from build123d import *

# Parameters (mm, degrees)
F0_R     = 5.25
F1_DEPTH = 5.5
F3_DEPTH = 6
F5_DEPTH = 6
F7_DEPTH = 6
F8_R     = 5


with BuildPart() as f1:
    # F0 (on Right) → F1 (new body)
    with BuildSketch(Plane.YZ):
        Polygon((76, -45), (76, 45), (-66, 45), (-66, 40), (-76, 40), (-76, -45), align=None)
        with Locations((-30, -25)):
            Circle(F0_R, mode=Mode.SUBTRACT)
        with Locations((-30, 26)):
            Circle(F0_R, mode=Mode.SUBTRACT)
    extrude(amount=F1_DEPTH)

    # F2 (on face) → F3 (join)
    with BuildSketch(Plane(origin=(0, 76, 0), x_dir=(-1, 0, 0), z_dir=(0, 1, 0))):
        with BuildLine():
            Line((110.5, 45), (0, 45))
            Line((0, 45), (0, -45))
            Line((0, -45), (81.5, -45))
            Line((81.5, -45), (81.5, -24.55))
            Line((81.5, -24.55), (40.525, -24.55))
            ThreePointArc((40.525, -24.55), (17, -1.025), (40.525, 22.5))
            Line((40.525, 22.5), (110.5, 22.5))
            Line((110.5, 22.5), (110.5, 45))
        make_face()
        with BuildLine():
            ThreePointArc((71.5, -30.525), (75.75, -34.775), (71.5, -39.025))
            Line((71.5, -39.025), (41.5, -39.025))
            ThreePointArc((41.5, -39.025), (37.25, -34.775), (41.5, -30.525))
            Line((41.5, -30.525), (71.5, -30.525))
        make_face(mode=Mode.SUBTRACT)
        with BuildLine():
            ThreePointArc((100.5, 38), (104.75, 33.75), (100.5, 29.5))
            Line((100.5, 29.5), (70.5, 29.5))
            ThreePointArc((70.5, 29.5), (66.25, 33.75), (70.5, 38))
            Line((70.5, 38), (100.5, 38))
        make_face(mode=Mode.SUBTRACT)
    extrude(amount=-F3_DEPTH)

    # F4 (on face) → F5 (join)
    with BuildSketch(Plane.XY.offset(45)):
        Polygon((0, -15), (0, 70), (-60, 70), align=None)
    extrude(amount=-F5_DEPTH)

    # F6 (on face) → F7 (join)
    with BuildSketch(Plane(origin=(0, 0, -45), x_dir=(1, 0, 0), z_dir=(0, 0, -1))):
        Polygon((-30, -70), (0, -70), (0, -10), align=None)
    extrude(amount=-F7_DEPTH)

    # F8
    f8_edges = [f1.edges().sort_by_distance(p)[0] for p in [
        (-110.5, 73, 45),
        (-110.5, 73, 22.5),
        (-81.5, 73, -24.55),
        (-81.5, 73, -45),
    ]]
    fillet(f8_edges, radius=F8_R)


solid = f1.part
Read the model definition and answer for the solid it produces. Units are mm, in the model's axes. A direction names the side the tool comes from. Coordinates: 2 decimals unless noted, no trailing zeros. Write each loop counter-clockwise with the first axis right and the second up, starting at its lowest first coordinate (ties: lowest second). Pieces come first, ordered by that corner, then holes. Notation, with made-up numbers: (22, 87) -> (53, 87) arc R30 cw to (53, 111) -> close; hole circle Ø11 at (32, 34.5). An arc over 180 degrees is marked (long way). Return JSON: item names as keys, results as strings.
(1) For a pull along X with two mould halves and no side action, classify faces 1 (the cylindrical face through (-75.75, 73.04, -34.68)), 2 (the cylindrical face through (2.71, -34.17, 22.81)), 3 (the cylindrical face through (-109, 72.96, 43.57)) as pulls with the +X half, pulls with the -X half, needs draft (parallel to the pull), parting line crosses it, or undercut.
Answers below:
{"face 1": "undercut", "face 2": "needs draft", "face 3": "pulls with the -X half"}
(2) The part is cut by section D-D on z = 4.5. Give the vertices of the cut face in (x, y).
Answers below:
{"outline": "(-17.66, 70) -> (0, 70) -> (0, -76) -> (5.5, -76) -> (5.5, 76) -> (-17.66, 76) -> close"}
(3) Consider line 1 along Z through (x, y) = (1.75, -30); line 2 along X through (y, z) = (3.5, -37.5); line 3 along Y through (x, z) = (-60, -41). Determine where each line is inside the solid, lowest interval first. Write a range as from..to.
Answers below:
{"line 1": "-45..-30.25, -19.75..20.75, 31.25..45", "line 2": "0..5.5", "line 3": "70..76"}
(4) Each of these flat-tipped pins is pushed along its axis until it touches: P1, Ø6, axis at x = 2, y = -73.5, coming from the +Z side; P2, Ø3, axis at x = -27.5, z = -21, coming from the -Y side; P3, Ø6.5, axis at y = 73.5, z = -34.5, coming from the -X side. Where does it stop, or does it pass through?
Answers below:
{"P1": "z = 40", "P2": "y = 70", "P3": "x = -81.5"}
(5) Which of the six approach directions +Z, -Z, +X, -X, +Y, -Y give full straight-line access (tool end or side, diameter ignored) to faces 4 (the flat face through (-59, 73, -24.55)), 5 (the flat face through (3, -71, 40)), 6 (the flat face through (0, -4, 1)), 7 (the flat face through (-57, 73, -39.025))?
Answers below:
{"face 4": "-X, +Y, -Y", "face 5": "+Z, +X, -X, -Y", "face 6": "-X, -Y", "face 7": "+Y, -Y"}
(6) The part is cut by section B-B on x = -57. Give the vertices of the cut face in (y, z) (3 decimals), then the cut area to 3 significant figures.
Answers below:
{"outline": "(65.75, 39) -> (70, 39) -> (70, 22.5) -> (76, 22.5) -> (76, 45) -> (65.75, 45) -> close; (70, -45) -> (76, -45) -> (76, -39.025) -> (70, -39.025) -> close; (70, -30.525) -> (76, -30.525) -> (76, -24.55) -> (70, -24.55) -> close", "area": "232 mm^2"}
(7) The part is cut by section C-C on y = 44. Give the vertices of the cut face in (x, z), then the cut area to 3 significant figures.
Answers below:
{"outline": "(-41.65, 39) -> (0, 39) -> (0, -39) -> (-17, -39) -> (-17, -45) -> (5.5, -45) -> (5.5, 45) -> (-41.65, 45) -> close", "area": "847 mm^2"}
(8) The part is cut by section A-A on x = -88. Give the vertices of the cut face in (y, z).
Answers below:
{"outline": "(70, 22.5) -> (76, 22.5) -> (76, 29.5) -> (70, 29.5) -> close; (70, 38) -> (76, 38) -> (76, 45) -> (70, 45) -> close"}
